Verification items for the finished model (mm, model axes). A direction names the side the tool comes from. Coordinates: 2 decimals unless noted, no trailing zeros. Order: outer loops, then holes, each group sorted by start corner. A loop starts at its lowest first (then second) coordinate and runs counter-clockwise, first axis right, second up. Notation, with made-up numbers: (-18, 9.5) -> (34, 9.5) arc R11 cw to (34, 19.5) -> close; hole circle Ø4 at (47, -26.75). An arc over 180 degrees is marked (long way). Answer as CSV lines item,"result".
```python
from build123d import *

# Parameters (mm, degrees)
SKETCH_W     = 20
SKETCH_H     = 20
SKETCH_R     = 1.6
PAD_DEPTH    = 8.5
POCKET_DEPTH = 3
FILLET_R     = 3


with BuildPart() as part:
    # Sketch → Pad (new body)
    with BuildSketch(Plane.XY):
        Rectangle(SKETCH_W, SKETCH_H)
        Circle(SKETCH_R, mode=Mode.SUBTRACT)
    extrude(amount=PAD_DEPTH)

    # Sketch001 (on Face7 of Pad) → Pocket (cut)
    with BuildSketch(Plane.XY.offset(8.5)):
        Polygon((1.616581, 2.8), (-1.616581, 2.8), (-3.233162, 0), (-1.616581, -2.8), (1.616581, -2.8), (3.233162, 0), align=None)
    extrude(amount=-POCKET_DEPTH, mode=Mode.SUBTRACT)

    # Fillet
    fillet_edges = [part.edges().sort_by_distance(p)[0] for p in [
        (10, -10, 4.25),
        (-10, -10, 4.25),
        (-10, 10, 4.25),
        (10, 10, 4.25),
    ]]
    fillet(fillet_edges, radius=FILLET_R)


solid = part.part
```
Item 1: Thickness scan on line 1 (X direction, y = 0, z = 2); line 2 (Y direction, x = -0.75, z = 3.5). Record the ranges inside material, lowest first.
Answer list:
line 1,"-10 to -1.6, 1.6 to 10"
line 2,"-10 to -1.41, 1.41 to 10"
Item 2: Section check C-C, the plane y = 8. Record the boundary of the cut face in (x, z).
Answer list:
outline,"(-9.83, 0) -> (9.83, 0) -> (9.83, 8.5) -> (-9.83, 8.5) -> close"
Item 3: Tool access check on faces 1 (the flat face through (-10, 0, 4)), 2 (the flat face through (2.414, -1.42, 7.021)). Record the directions out of +Z, -Z, +X, -X, +Y, -Y that give a thin tool (end or side, any length) a straight path to the whole face; none if there is none.
Answer list:
face 1,"+Z, -Z, -X, +Y, -Y"
face 2,"+Z"
Item 4: Section check B-B, the plane x = 0. Record the boundary of the cut face in (y, z).
Answer list:
outline,"(-10, 0) -> (-1.6, 0) -> (-1.6, 5.5) -> (-2.8, 5.5) -> (-2.8, 8.5) -> (-10, 8.5) -> close; (1.6, 0) -> (10, 0) -> (10, 8.5) -> (2.8, 8.5) -> (2.8, 5.5) -> (1.6, 5.5) -> close"
Item 5: Section check A-A, the plane z = 2.25. Record the boundary of the cut face in (x, y), plus the area to 3 significant figures.
Answer list:
outline,"(-10, -7) arc R3 ccw to (-7, -10) -> (7, -10) arc R3 ccw to (10, -7) -> (10, 7) arc R3 ccw to (7, 10) -> (-7, 10) arc R3 ccw to (-10, 7) -> close; hole circle Ø3.2 at (0, 0)"
area,"384 mm2"
